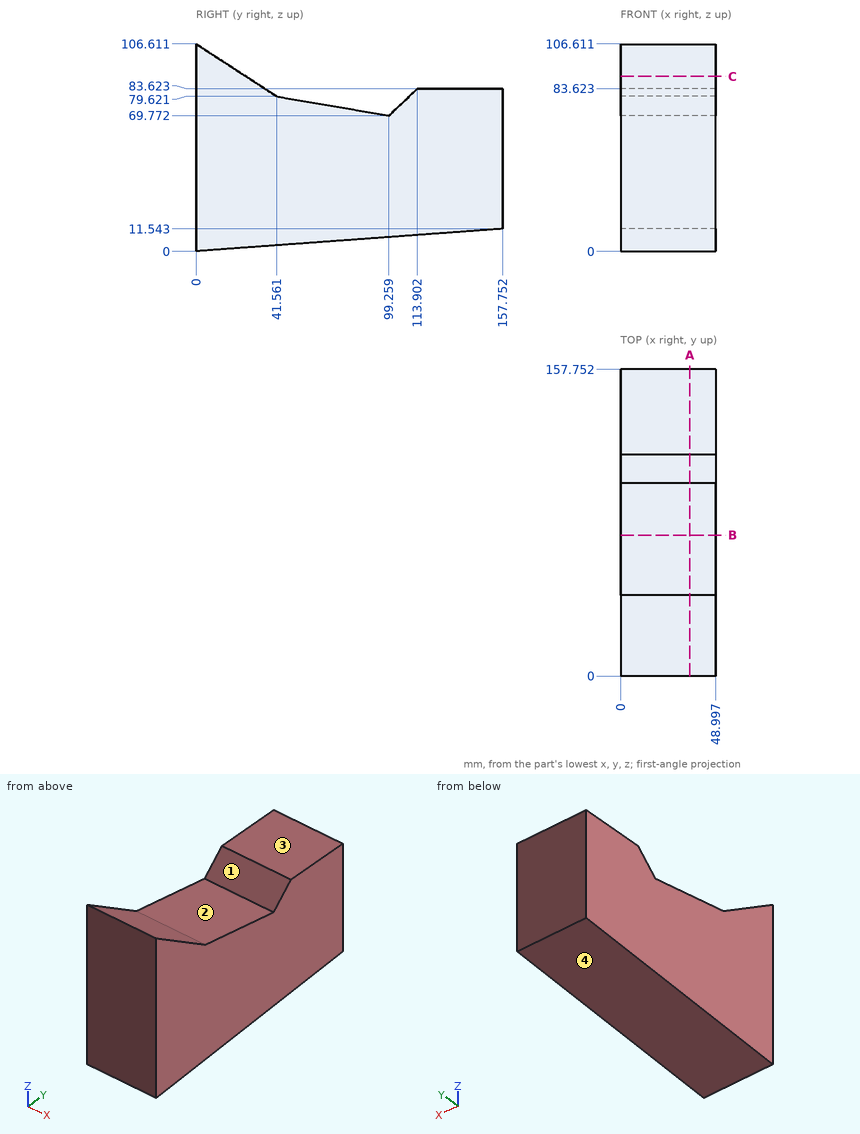
Answer from the drawing. Dimensions are ordinates in mm from the lowest x, y and z of the part. Give positions to 0.01 mm unless a question says otherwise; leave off trailing zeros. Order: outer loops, then holes, each group sorted by start corner. A loop starts at its lowest first (then second) coordinate and runs counter-clockwise, first axis right, second up.
Item 1: For a pull along Y with two mould halves and no side action, classify the marked faces 1, 2, 3 and 4 as pulls with the +Y half, pulls with the -Y half, needs draft (parallel to the pull), parting line crosses it, or undercut.
From the geometry:
face 1: undercut
face 2: undercut
face 3: needs draft
face 4: pulls with the +Y half
Item 2: The part is cut by section B-B, the plane y = 72.5. Give the vertices of the cut face in (x, z) (1 decimal).
From the geometry:
outline: (0, 5.3) - (49, 5.3) - (49, 74.3) - (0, 74.3) - close
Item 3: The part is cut by section A-A, the plane x = 35.5. Give the vertices of the cut face in (y, z), and give its area (3 significant figures).
From the geometry:
outline: (0, 0) - (157.75, 11.54) - (157.75, 83.62) - (113.9, 83.62) - (99.26, 69.77) - (41.56, 79.62) - (0, 106.61) - close
area: 12,100 mm2
Item 4: Find the intervals of material crossed by probe 1 along Y at (x, z) = (17, 94) (1 decimal); probe 2 along Z at (x, y) = (38, 17) (1 decimal); probe 3 along Z at (x, y) = (23.5, 109) (1 decimal), in increasing order.
From the geometry:
probe 1: y = 0 to 19.4
probe 2: z = 1.2 to 95.6
probe 3: z = 8 to 79
Item 5: Given pin 1 Ø8 at (x, y) = (34.5, 138) entering from +Z; pin 2 Ø10 at (x, y) = (7.5, 118) entering from -Z; pin 3 Ø1 at (x, y) = (7, 62.5) entering from +Z, each flat-ended and moving along its own axis, determine where each tip first touches the part or whether it passes through.
From the geometry:
pin 1: stops at z = 83.62
pin 2: stops at z = 8.27
pin 3: stops at z = 76.13
Item 6: The part is cut by section C-C, the plane z = 90. Give the vertices of the cut face in (x, y), and give its area (3 significant figures).
From the geometry:
outline: (0, 0) - (49, 0) - (49, 25.58) - (0, 25.58) - close
area: 1,250 mm2
